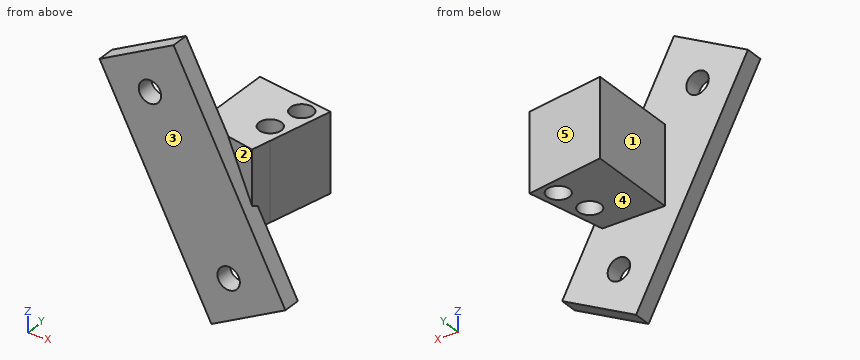
from build123d import *

# Parameters (mm, degrees)
SKETCH2_R           = 3.175
BOSS_EXTRUDE1_DEPTH = 22.098
SKETCH3_W           = 8.89
SKETCH3_H           = 22.098
BOSS_EXTRUDE2_DEPTH = 7.62
SKETCH4_R           = 3.175
BOSS_EXTRUDE3_DEPTH = 5.0531014
BOSS_EXTRUDE4_DEPTH = 22.098
CUT_EXTRUDE1_DEPTH  = 126.746
BOSS_EXTRUDE6_REACH = 111.16
SKETCH8_W           = 22.098
SKETCH8_H           = 5.750865106


with BuildPart() as part:
    # Sketch2 → Boss-Extrude1 (new body)
    # profile 1 of 2: a face of its own
    with BuildSketch(Plane.XY):
        with BuildLine():
            Line((-633.396746705, 209.866473294), (-629.456250373, 228.608305414))
            Line((-629.456250373, 228.608305414), (-640.203126947, 230.867851197))
            ThreePointArc((-640.203126947, 230.867851197), (-642.751451447, 226.300988286), (-641.845462116, 221.150320569))
            ThreePointArc((-641.845462116, 221.150320569), (-644.490547106, 217.002439965), (-644.037989982, 212.103809529))
            Line((-644.037989982, 212.103809529), (-633.396746705, 209.866473294))
        make_face()
        with Locations(Location((-637.11116423, 215.213960129, 0), (0, 0, 180))):
            Circle(SKETCH2_R, mode=Mode.SUBTRACT)
        with Locations(Location((-635.053635704, 225, 0), (0, 0, 180))):
            Circle(SKETCH2_R, mode=Mode.SUBTRACT)
    # profile 2 of 2: a face of its own
    with BuildSketch(Plane.XY):
        with BuildLine():
            ThreePointArc((-641.845462116, 221.150320569), (-642.751451447, 226.300988286), (-640.203126947, 230.867851197))
            Line((-640.203126947, 230.867851197), (-646.417262265, 232.174381811))
            Line((-646.417262265, 232.174381811), (-650.357758597, 213.432549691))
            Line((-650.357758597, 213.432549691), (-644.037989982, 212.103809529))
            ThreePointArc((-644.037989982, 212.103809529), (-644.490547106, 217.002439965), (-641.845462116, 221.150320569))
        make_face()
    extrude(amount=BOSS_EXTRUDE1_DEPTH)

    # Sketch3 → Boss-Extrude2 (add)
    with BuildSketch(Plane(origin=(15.442364745, 73.44714554, 0), x_dir=(0.9786039871389689, -0.20575285260650172, 0), z_dir=(-0.20575285260650172, -0.9786039871389689, 0))):
        with Locations((-675.912051568, 11.049)):
            Rectangle(SKETCH3_W, SKETCH3_H)
    extrude(amount=BOSS_EXTRUDE2_DEPTH)

    # Sketch4 → Boss-Extrude3 (add)
    with BuildSketch(Plane(origin=(0, 205.975587309, 0), x_dir=(1, 0, 0), z_dir=(0, 1, 0))):
        Polygon((-643.78094836, 26.639989184), (-675.455245779, -34.187268547), (-654.503634783, -45.097304324), (-622.829337364, 15.729953406), align=None)
        with Locations(Location((-638.898775927, 12.642774556, 0), (0, 0, 270))):
            Circle(SKETCH4_R, mode=Mode.SUBTRACT)
        with Locations(Location((-661.188096333, -30.161591995, 0), (0, 0, 270))):
            Circle(SKETCH4_R, mode=Mode.SUBTRACT)
    extrude(amount=-BOSS_EXTRUDE3_DEPTH)

    # Sketch5 → Boss-Extrude4 (add)
    with BuildSketch(Plane.XY.offset(22.098)):
        Polygon((-651.925595334, 205.975587309), (-651.925595334, 232.199360665), (-646.417262265, 232.174381811), align=None)
    extrude(amount=-BOSS_EXTRUDE4_DEPTH)

    # Sketch6 → Cut-Extrude1 (cut)
    with BuildSketch(Plane(origin=(0, 0, 0), x_dir=(-1, 0, 0), z_dir=(0, 0, -1))):
        Polygon((629.456250373, 228.608305414), (651.925595334, 232.199360665), (646.417262265, 232.174381811), align=None)
    extrude(amount=-CUT_EXTRUDE1_DEPTH, mode=Mode.SUBTRACT)

    # Boss-Extrude6: up to this face of the body (flat: up to its plane)
    boss_extrude6_end = Plane(part.part.faces().sort_by_distance((-642.249597602, 208.78949707, 11.049))[0])
    # Sketch8 → Boss-Extrude6 (add, up to the picked face)
    with BuildSketch(Plane(origin=(-648.83911145, 136.419327755, 0), x_dir=(0, 0, -1), z_dir=(0.9786039871389688, -0.20575285260650203, 0)), mode=Mode.PRIVATE) as boss_extrude6_sk1:
        with Locations((-11.049, 72.177547513)):
            Rectangle(SKETCH8_W, SKETCH8_H)
    boss_extrude6_tool1 = split(extrude(boss_extrude6_sk1.sketch, amount=-BOSS_EXTRUDE6_REACH, mode=Mode.PRIVATE), bisect_by=boss_extrude6_end, keep=Keep.BOTH, mode=Mode.PRIVATE)
    add(boss_extrude6_tool1.solids().sort_by(Axis((-633.988375, 207.052564, 11.049), (-0.9786039871389688, 0.20575285260650203, 0)))[0])


solid = part.part
Can you work these out from the model? Positions are in its coordinate system, mm. Face numbers are marked on the shaded views. A direction names the side the tool comes from. Give positions to 0.01 mm unless a question says otherwise; leave off trailing zeros. Loops run counter-clockwise (first coordinate to the right, second up) from the corner with the lowest first, then second, coordinate; pieces in that order, holes last. Notation, with made-up numbers: (78.5, -5) -> (94.5, -5) arc R25 ccw to (94.5, 23) -> close; hole circle Ø4 at (39, 56). An arc over 180 degrees is marked (long way). Write item = value, one per line.
1) Will these pins go through, and if not, where does the flat tip stop? pin 1 (1 mm diameter, centred on x = -668.5, y = 207.5, fed in from -Z); pin 2 (6.5 mm diameter, centred on x = -635.5, y = 224, fed in from +Z); pin 3 (11 mm diameter, centred on x = -643.5, y = 219, fed in from -Z); pin 4 (2 mm diameter, centred on y = 205, z = 3.5, fed in from +X).
Check result:
pin_1 = through
pin_2 = 22.1
pin_3 = 0
pin_4 = -632.32
2) Suppose I cut it at B-B on z = 11. Write out the boundary of the cut face in (x, y) (3 decimals), then the cut area to 3 significant figures.
Check result:
outline = (-663.381, 200.922) -> (-636.748, 200.922) -> (-636.748, 204.695) -> (-634.58, 204.239) -> (-629.456, 228.608) -> (-651.926, 232.199) -> (-651.926, 205.976) -> (-663.381, 205.976) -> close; hole circle Ø6.35 at (-637.111, 215.214); hole circle Ø6.35 at (-635.054, 225)
area = 570 mm2
3) For the marked faces 4 and 5, which set-ups out of +Z, -Z, +X, -X, +Y, -Y let a thin tool reach every point of the face, with its end or its side?
Check result:
face_4 = -Z, +X, -X, +Y
face_5 = +Z, -Z, +X, +Y
4) Suppose I cut it at C-C on x = -660. Write out the boundary of the cut face in (y, z), then the cut area to 3 significant figures.
Check result:
outline = (200.92, 4.51) -> (205.98, 4.51) -> (205.98, 27.22) -> (200.92, 27.22) -> close; (200.92, 33.11) -> (205.98, 33.11) -> (205.98, 42.24) -> (200.92, 42.24) -> close
area = 161 mm2
5) Suppose I cut it at D-D on z = 37. Write out the boundary of the cut face in (x, y), then the cut area to 3 significant figures.
Check result:
outline = (-670.05, 200.92) -> (-650.29, 200.92) -> (-650.29, 205.98) -> (-670.05, 205.98) -> close
area = 99.9 mm2
6) I need wall thicknesses on L1, parallel to Z at x = -638, y = 223; L2, parallel to Y at x = -636, z = -3; L3, parallel to Y at x = -636, z = 12.5. Which ranges of each line are inside material? Lowest first, please. Write a range as from..to.
Check result:
L1 = 0..22.1
L2 = 200.92..205.98
L3 = 204.54..212.24, 218.19..221.97, 228.03..229.65
7) Suppose I cut it at A-A on y = 225. Write out the boundary of the cut face in (x, z).
Check result:
outline = (-651.93, 0) -> (-638.23, 0) -> (-638.23, 22.1) -> (-651.93, 22.1) -> close; (-631.88, 0) -> (-630.21, 0) -> (-630.21, 22.1) -> (-631.88, 22.1) -> close
8) Thinking about a two-plate mould opening in X: for the marked faces 1, 2 and 3, which applies, released by +X, released by -X, zero draft, split by the parting line, or undercut?
Check result:
face_1 = released by -X
face_2 = undercut
face_3 = zero draft
